from build123d import *

# Parameters (mm, degrees)
BOSS_EXTRUDE1_DEPTH = 127
SKETCH3_R           = 25
BOSS_EXTRUDE2_DEPTH = 20
SKETCH4_R           = 22
CUT_EXTRUDE2_DEPTH  = 148


with BuildPart() as part:
    # Sketch1 → Boss-Extrude1 (new body)
    with BuildSketch(Plane(origin=(0, 0, 0), x_dir=(1, 0, 0), z_dir=(0, 1, 0))):
        with BuildLine():
            Line((-30, 0), (-30, -30))
            Line((-30, -30), (30, -30))
            Line((30, -30), (30, 0))
            ThreePointArc((30, 0), (0, 30), (-30, 0))
        make_face()
    extrude(amount=BOSS_EXTRUDE1_DEPTH)

    # Sketch3 → Boss-Extrude2 (add)
    with BuildSketch(Plane(origin=(0, 0, 0), x_dir=(-1, 0, 0), z_dir=(0, -1, 0))):
        Circle(SKETCH3_R)
    extrude(amount=BOSS_EXTRUDE2_DEPTH)

    # Sketch4 → Cut-Extrude2 (cut, through all)
    with BuildSketch(Plane(origin=(0, -20, 0), x_dir=(-1, 0, 0), z_dir=(0, -1, 0))):
        Circle(SKETCH4_R)
    extrude(amount=-CUT_EXTRUDE2_DEPTH, mode=Mode.SUBTRACT)


solid = part.part
Geometry check sheet. Reference: the model listing, model coordinates, mm. A direction names the side the tool comes from. Round coordinates to 2 decimals unless told otherwise and drop trailing zeros. Order: outer loops, then holes, each group sorted by start corner. A loop starts at its lowest first (then second) coordinate and runs counter-clockwise, first axis right, second up. Notation, with made-up numbers: M 83,-25 L 141,-25 A37 cw 141,12 Z; hole C -12,24 d1. An arc over 180 degrees is marked long. Answer in a Markdown table with one row per item. Add a question column.
Item 1: Sectioned sample at A-A, the plane x = 0. Enter the section's corners in (y, z), plus the area to 3 significant figures.
Item 2: Depth check by flat-ended pin: pin 1 Ø3 at (x, z) = (21, -17) entering from -Y; pin 2 Ø6 at (x, y) = (11.5, -1.5) entering from -Z; pin 3 Ø1.5 at (x, y) = (15, 91.5) entering from -Z. Enter the tip coordinate at first touch or a pass-through.
Item 3: Sectioned sample at C-C, the plane y = -3. Enter the section's corners in (x, z).
Item 4: Sectioned sample at D-D, the plane z = 23.5. Enter the section's corners in (x, y), plus the area to 3 significant figures.
Item 5: Draft check along X on faces 1 (the face through (-23.846, -9.86, -7.509)), 2 (the face through (-30, 63, 15)), 3 (the face through (4.769, 52.471, 21.477)), 4 (the face through (0, 63, 30)). Enter one of: released by +X, released by -X, zero draft, split by the parting line, or undercut.
Item 6: Material ranges on L1, parallel to X at y = 32, z = 0; L2, parallel to Y at x = -17.5, z = 19.5, recorded low to high. Write a range as [from, to].
Item 7: Sectioned sample at B-B, the plane z = -2. Enter the section's corners in (x, y), plus the area to 3 significant figures.
Item 8: Set-up check for faces 5 (the face through (-9, 0, 24)), 6 (the face through (30, 63, 15)): record each of +Z, -Z, +X, -X, +Y, -Y from which the full face is reachable in a straight line by a thin tool's end or side.
Filled in:
| question | item | result |
|---|---|---|
| 1 | outline | M -20,-25 L 0,-25 L 0,-30 L 127,-30 L 127,-22 L -20,-22 Z; M -20,22 L 127,22 L 127,30 L 0,30 L 0,25 L -20,25 Z |
| 1 | area | 2,150 mm² |
| 2 | pin 1 | stops at y = 0 |
| 2 | pin 2 | stops at z = -28.65 |
| 2 | pin 3 | stops at z = -26.4 |
| 3 | outline | C 0,0 d50; hole C 0,0 d44 |
| 4 | outline | M -30,0 L -8.53,0 L -8.53,-20 L 8.53,-20 L 8.53,0 L 30,0 L 30,127 L -30,127 Z |
| 4 | area | 7,960 mm² |
| 5 | face 1 | split by the parting line |
| 5 | face 2 | released by -X |
| 5 | face 3 | undercut |
| 5 | face 4 | zero draft |
| 6 | L1 | x = [-30, -22], [22, 30] |
| 6 | L2 | y = [0, 127] |
| 7 | outline | M -29.93,0 L -24.92,0 L -24.92,-20 L -21.91,-20 L -21.91,127 L -29.93,127 Z; M 21.91,-20 L 24.92,-20 L 24.92,0 L 29.93,0 L 29.93,127 L 21.91,127 Z |
| 7 | area | 2,160 mm² |
| 8 | face 5 | -Y |
| 8 | face 6 | +Z, -Z, +X, +Y, -Y |
